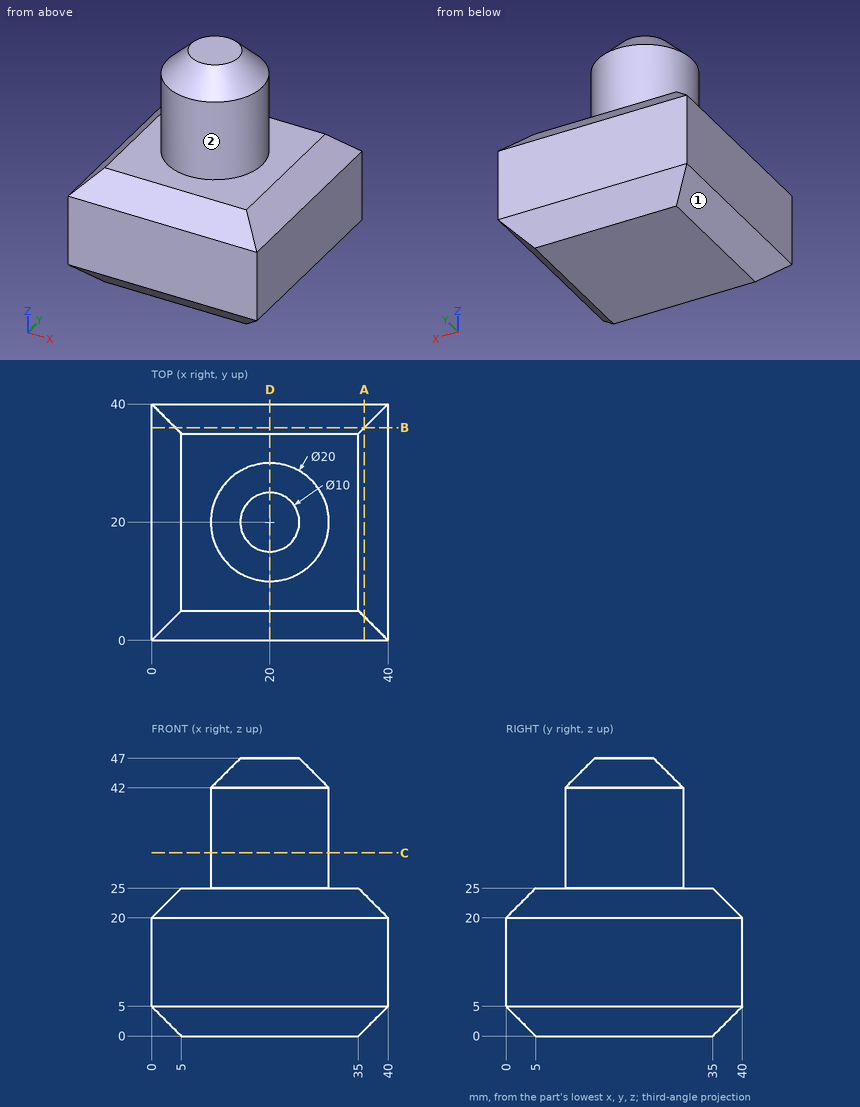
Job drawing, mm, ordinate dimensions from the low corner. One solid piece. A direction names the side the tool comes from. Round coordinates to 2 decimals unless told otherwise and drop trailing zeros. Write each loop counter-clockwise with the first axis right and the second up, starting at its lowest first coordinate (ties: lowest second). Pieces come first, ordered by that corner, then holes. Notation, with made-up numbers: M -19,26 L 12,26 A7 cw 12,33 Z; hole C 53.5,86 d3. An arc over 180 degrees is marked long. Return JSON: item names as keys, results as strings. Group by question number.
(1) Pin check, flat tips, straight feed: pin 1 Ø2 at (x, y) = (26.5, 7) entering from +Z; pin 2 Ø6 at (y, z) = (24.5, 33.5) entering from +X; pin 3 Ø4 at (y, z) = (28.5, 42) entering from -X. Stop position of each tip, or through.
(2) Saw through at D-D on x = 20. Write the cut outline in (y, z), then the cut area to 4 significant figures.
(3) Saw through at A-A on x = 36. Write the cut outline in (y, z), then the cut area to 3 significant figures.
(4) Which spindle directions (+Z, -Z, +X, -X, +Y, -Y) get a long thin tool onto all of the face, cutting with end or side? Do the marked faces 1 and 2. Say none if no direction does.
(5) Drill centre lines: probe 1 along Z at (x, y) = (9, 32); probe 2 along Z at (x, y) = (13, 15); probe 3 along X at (y, z) = (36, 22). Where is each one in solid material? Low to high.
(6) Saw through at C-C on z = 31. Write the cut outline in (x, y).
Returned:
{
 "1": {"pin 1": "z = 25", "pin 2": "x = 29.89", "pin 3": "x = 12.4"},
 "2": {"outline": "M 0,5 L 5,0 L 35,0 L 40,5 L 40,20 L 35,25 L 30,25 L 30,42 L 25,47 L 15,47 L 10,42 L 10,25 L 5,25 L 0,20 Z", "area": "1,365 mm²"},
 "3": {"outline": "M 0,5 L 4,1 L 36,1 L 40,5 L 40,20 L 36,24 L 4,24 L 0,20 Z", "area": "888 mm²"},
 "4": {"face 1": "-Z, -X, +Y, -Y", "face 2": "+Z"},
 "5": {"probe 1": "0 to 25", "probe 2": "0 to 43.4", "probe 3": "2 to 38"},
 "6": {"outline": "C 20,20 d20"}
}
